Build history of the part. All positions in model axes, mm. Give positions to 0.01 mm unless a question says otherwise; leave off trailing zeros. Loops run counter-clockwise (first coordinate to the right, second up) from the corner with the lowest first, then second, coordinate; pieces in that order, holes last. Notation, with made-up numbers: M 63,13 L 111,13 A18 cw 111,28 Z; hole C 74,39 d7. An arc over 180 degrees is marked long. Answer as a JSON object with one key per item and string values. Group by question number.
1. Drop flat-ended pins along their axis: pin 1 Ø5 at (x, z) = (2.5, 6.5) entering from -Y; pin 2 Ø0.8 at (y, z) = (1, -6.5) entering from -X; pin 3 Ø0.8 at (x, y) = (-15.5, 0.5) entering from -Z. Give the stop position or say it passes through.
2. Slice it at A-A (y = 1). List the corners of the cut face in (x, z).
3. Slice it at C-C (x = 17). List the corners of the cut face in (y, z).
4. Drill centre lines: line 1 along Z through (x, y) = (-22, 0.2); line 2 along X through (y, z) = (0.3, 7.75). Where is each one in solid material? Low to high. Write a range as [from, to].
5. Slice it at B-B (z = -6). List the corners of the cut face in (x, y).
from build123d import *

# Parameters (mm, degrees)
SKETCH1_W           = 49
SKETCH1_H           = 11
BOSS_EXTRUDE1_DEPTH = 1.5
SKETCH2_W           = 5
SKETCH2_H           = 3
BOSS_EXTRUDE2_DEPTH = 1.5
SKETCH3_W           = 5
SKETCH3_H           = 3
BOSS_EXTRUDE3_DEPTH = 1.5


with BuildPart() as part:
    # Sketch1 → Boss-Extrude1 (new body)
    with BuildSketch(Plane(origin=(0, 0, 0), x_dir=(1, 0, 0), z_dir=(0, 1, 0))):
        Rectangle(SKETCH1_W, SKETCH1_H)
    extrude(amount=BOSS_EXTRUDE1_DEPTH)

    # Sketch2 → Boss-Extrude2 (add)
    with BuildSketch(Plane(origin=(0, 1.5, 0), x_dir=(1, 0, 0), z_dir=(0, 1, 0))):
        with Locations((0, 7)):
            Rectangle(SKETCH2_W, SKETCH2_H)
    extrude(amount=-BOSS_EXTRUDE2_DEPTH)

    # Sketch3 → Boss-Extrude3 (add)
    with BuildSketch(Plane(origin=(0, 1.5, 0), x_dir=(1, 0, 0), z_dir=(0, 1, 0))):
        with Locations((0, -7)):
            Rectangle(SKETCH3_W, SKETCH3_H)
    extrude(amount=-BOSS_EXTRUDE3_DEPTH)


solid = part.part
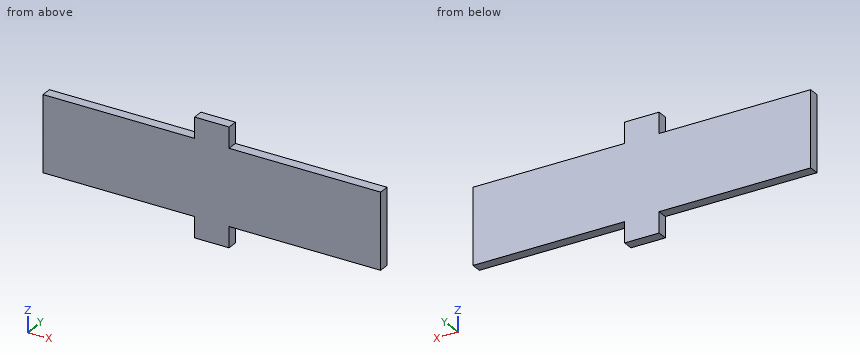
Established:
{
 "1": {"pin 1": "stops at y = 0", "pin 2": "stops at x = -2.5", "pin 3": "stops at z = -5.5"},
 "2": {"outline": "M -24.5,-5.5 L -2.5,-5.5 L -2.5,-8.5 L 2.5,-8.5 L 2.5,-5.5 L 24.5,-5.5 L 24.5,5.5 L 2.5,5.5 L 2.5,8.5 L -2.5,8.5 L -2.5,5.5 L -24.5,5.5 Z"},
 "3": {"outline": "M 0,-5.5 L 1.5,-5.5 L 1.5,5.5 L 0,5.5 Z"},
 "4": {"line 1": "z = [-5.5, 5.5]", "line 2": "x = [-2.5, 2.5]"},
 "5": {"outline": "M -2.5,0 L 2.5,0 L 2.5,1.5 L -2.5,1.5 Z"}
}
